Could you check a few things on this model? Use its own coordinates, in mm. Give positions to 0.01 mm unless a question says otherwise; leave off trailing zeros. Order: outer loops, then holes, each group sorted by start corner. A loop starts at its lowest first (then second) coordinate and runs counter-clockwise, first axis right, second up. Notation, with made-up numbers: M 20,48 L 28,48 A16 ccw 28,58 Z; hole C -11,-4 d7. An arc over 180 degrees is marked long. Use a Markdown table: item, result. Add a question column.
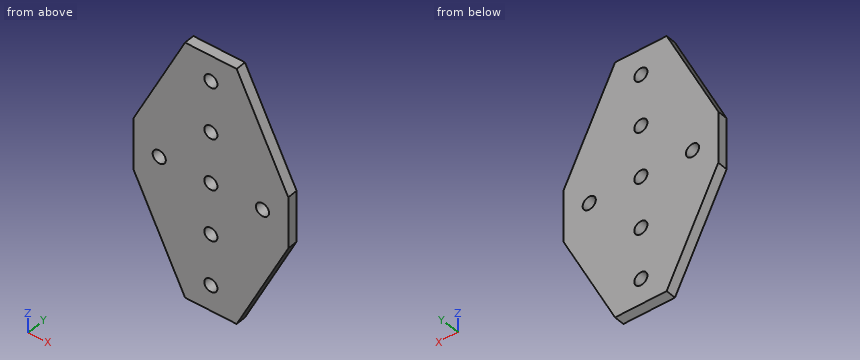
```python
from build123d import *

# Parameters (mm, degrees)
SKETCH1_R           = 2.55
BOSS_EXTRUDE1_DEPTH = 4


with BuildPart() as part:
    # Sketch1 → Boss-Extrude1 (new body)
    with BuildSketch(Plane(origin=(0, 0, 0), x_dir=(1, 0, 0), z_dir=(0, 1, 0))):
        Polygon((30, -10), (10, -50), (-10, -50), (-30, -10), (-30, 10), (-10, 50), (10, 50), (30, 10), align=None)
        with Locations((0, 20)):
            Circle(SKETCH1_R, mode=Mode.SUBTRACT)
        with Locations((0, 40)):
            Circle(SKETCH1_R, mode=Mode.SUBTRACT)
        Circle(SKETCH1_R, mode=Mode.SUBTRACT)
        with Locations((0, -20)):
            Circle(SKETCH1_R, mode=Mode.SUBTRACT)
        with Locations((0, -40)):
            Circle(SKETCH1_R, mode=Mode.SUBTRACT)
        with Locations((-20, 0)):
            Circle(SKETCH1_R, mode=Mode.SUBTRACT)
        with Locations((20, 0)):
            Circle(SKETCH1_R, mode=Mode.SUBTRACT)
    extrude(amount=BOSS_EXTRUDE1_DEPTH)


solid = part.part
```
1) Suppose I cut it at A-A on x = 0. Please give me the cut outline in (y, z).
2) Suppose I cut it at D-D on z = 0. Please give me the cut outline in (x, y), and give its area (3 significant figures).
3) Please list where these lines run through material, in increasing order: line 1 (Z direction, x = 0, y = 1.2); line 2 (X direction, y = 1.2, z = 0); line 3 (Z direction, x = -1, y = 1). Write a range as from..to.
4) Suppose I cut it at B-B on x = 20. Please give me the cut outline in (y, z).
5) For pin 1 (1 mm diameter, centred on x = 17, y = 2.5, fed in from +Z); pin 2 (2 mm diameter, centred on x = 14, y = 1, fed in from +Z); pin 3 (4.5 mm diameter, centred on x = 0, z = -20, fed in from +Y), each with a flat end and sliding along its axis, tell me the tip position at first contact or that it passes through.
6) Suppose I cut it at C-C on z = -20. Please give me the cut outline in (x, y), and give its area (3 significant figures).
Values found:
| question | item | result |
|---|---|---|
| 1 | outline | M 0,-50 L 4,-50 L 4,-42.55 L 0,-42.55 Z; M 0,-37.45 L 4,-37.45 L 4,-22.55 L 0,-22.55 Z; M 0,-17.45 L 4,-17.45 L 4,-2.55 L 0,-2.55 Z; M 0,2.55 L 4,2.55 L 4,17.45 L 0,17.45 Z; M 0,22.55 L 4,22.55 L 4,37.45 L 0,37.45 Z; M 0,42.55 L 4,42.55 L 4,50 L 0,50 Z |
| 2 | outline | M -30,0 L -22.55,0 L -22.55,4 L -30,4 Z; M -17.45,0 L -2.55,0 L -2.55,4 L -17.45,4 Z; M 2.55,0 L 17.45,0 L 17.45,4 L 2.55,4 Z; M 22.55,0 L 30,0 L 30,4 L 22.55,4 Z |
| 2 | area | 179 mm^2 |
| 3 | line 1 | z = -50..-42.55, -37.45..-22.55, -17.45..-2.55, 2.55..17.45, 22.55..37.45, 42.55..50 |
| 3 | line 2 | x = -30..-22.55, -17.45..-2.55, 2.55..17.45, 22.55..30 |
| 3 | line 3 | z = -50..-42.35, -37.65..-22.35, -17.65..-2.35, 2.35..17.65, 22.35..37.65, 42.35..50 |
| 4 | outline | M 0,-30 L 4,-30 L 4,-2.55 L 0,-2.55 Z; M 0,2.55 L 4,2.55 L 4,30 L 0,30 Z |
| 5 | pin 1 | stops at z = 37 |
| 5 | pin 2 | stops at z = 44 |
| 5 | pin 3 | passes through |
| 6 | outline | M -25,0 L -2.55,0 L -2.55,4 L -25,4 Z; M 2.55,0 L 25,0 L 25,4 L 2.55,4 Z |
| 6 | area | 180 mm^2 |
